Geometry check sheet. Reference: the model listing, model coordinates, mm. A direction names the side the tool comes from. Give positions to 0.01 mm unless a question says otherwise; leave off trailing zeros. Loops run counter-clockwise (first coordinate to the right, second up) from the corner with the lowest first, then second, coordinate; pieces in that order, holes last. Notation, with made-up numbers: (63, -38.75) -> (70, -38.75) arc R19 cw to (70, -31.75) -> close; hole circle Ø6 at (-18.5, -19.5). An arc over 180 degrees is marked (long way). Answer as a JSON object with one key per item and string values.
from build123d import *

# Parameters (mm, degrees)
FILLET1_R     = 2.5
CHAMFER1_SIZE = 1


with BuildPart() as part:
    # Sketch1 → Revolve1 (revolve)
    with BuildSketch(Plane.XY):
        Polygon((0, 0), (0, 10), (30, 10), (30, 12.5), (55, 12.5), (55, 15), (65, 15), (70, 10), (100, 10), (100, 0), align=None)
    revolve(axis=Axis((100, 0, 0), (-1, 0, 0)))

    # Fillet1
    fillet1_edges = [part.edges().sort_by_distance(p)[0] for p in [
        (30, -10, 0),
        (55, -12.5, 0),
    ]]
    fillet(fillet1_edges, radius=FILLET1_R - 0.0001)  # a hair under: the kernel refuses the full size

    # Chamfer1
    chamfer1_edges = [part.edges().sort_by_distance(p)[0] for p in [
        (0, -10, 0),
        (100, -10, 0),
    ]]
    chamfer(chamfer1_edges, length=CHAMFER1_SIZE)


solid = part.part
1) Tool access check on faces 1 (the face through (84.7, -2.17, 9.76)), 2 (the face through (0, 0, 0)), 3 (the face through (41.408, 11.923, -3.755)). Record the directions out of +Z, -Z, +X, -X, +Y, -Y that give a thin tool (end or side, any length) a straight path to the whole face; none if there is none.
Geometry check:
{"face 1": "+X", "face 2": "+Z, -Z, -X, +Y, -Y", "face 3": "-X"}
2) Material ranges on line 1 along Y through (x, z) = (40.5, 7.5); line 2 along X through (y, z) = (0, 9); line 3 along Z through (x, y) = (93, -8.5), recorded low to high. Write a range as from..to.
Geometry check:
{"line 1": "y = -10..10", "line 2": "x = 0..100", "line 3": "z = -5.27..5.27"}
3) Depth check by flat-ended pin: P1, Ø3, axis at x = 63, y = -11, coming from the +Z side; P2, Ø4, axis at x = 48, y = 10, coming from the +Z side; P3, Ø12, axis at x = 34, z = -12, coming from the +Y side. Enter the tip coordinate at first touch or a pass-through.
Geometry check:
{"P1": "stops at z = 11.61", "P2": "stops at z = 9.6", "P3": "stops at y = 10.97"}
4) Section check D-D on x = 45. Record the cut outline in (y, z), plus the area to 3 significant figures.
Geometry check:
{"outline": "circle Ø25 at (0, 0)", "area": "491 mm2"}
5) Section check C-C on x = 82. Record the cut outline in (y, z), plus the area to 3 significant figures.
Geometry check:
{"outline": "circle Ø20 at (0, 0)", "area": "314 mm2"}
